from build123d import *

# Parameters (mm, degrees)
SKETCH1_R           = 39.751
BOSS_EXTRUDE1_DEPTH = 103.124
SKETCH2_R           = 17.4625
BOSS_EXTRUDE2_DEPTH = 2.54
SKETCH3_R           = 6.35
BOSS_EXTRUDE3_DEPTH = 41.91
BOSS_EXTRUDE4_START = 14.224
SKETCH4_R           = 6.35
BOSS_EXTRUDE4_DEPTH = 14.224
SKETCH5_R           = 1.999996
CUT_EXTRUDE1_DEPTH  = 6.858


with BuildPart() as part:
    # Sketch1 → Boss-Extrude1 (new body)
    with BuildSketch(Plane(origin=(0, 0, 0), x_dir=(0, 0, -1), z_dir=(1, 0, 0))):
        Circle(SKETCH1_R)
    extrude(amount=BOSS_EXTRUDE1_DEPTH)

    # Sketch2 → Boss-Extrude2 (add)
    with BuildSketch(Plane(origin=(103.124, 0, 0), x_dir=(0, 0, -1), z_dir=(1, 0, 0))):
        Circle(SKETCH2_R)
    extrude(amount=BOSS_EXTRUDE2_DEPTH)

    # Sketch3 → Boss-Extrude3 (add)
    with BuildSketch(Plane(origin=(105.664, 0, 0), x_dir=(0, 0, -1), z_dir=(1, 0, 0))):
        Circle(SKETCH3_R)
    extrude(amount=BOSS_EXTRUDE3_DEPTH)

    # Sketch4 → Boss-Extrude4 (add)
    with BuildSketch(Plane.ZY.offset(BOSS_EXTRUDE4_START)):
        with Locations(Location((0, 0, 0), (0, 0, 180))):
            Circle(SKETCH4_R)
    extrude(amount=-BOSS_EXTRUDE4_DEPTH)

    # Sketch5 → Cut-Extrude1 (cut)
    with BuildSketch(Plane(origin=(103.124, 0, 0), x_dir=(0, 0, -1), z_dir=(1, 0, 0))):
        with Locations((-14.882420075, 20.086004442)):
            Circle(SKETCH5_R)
        with Locations((20.086004442, 14.882420075)):
            Circle(SKETCH5_R)
        with Locations((14.882420075, -20.086004442)):
            Circle(SKETCH5_R)
        with Locations((-20.086004442, -14.882420075)):
            Circle(SKETCH5_R)
    extrude(amount=-CUT_EXTRUDE1_DEPTH, mode=Mode.SUBTRACT)


solid = part.part
Check sheet for the modelled part. Datum: model origin and axes. Units: mm. A direction names the side the tool comes from. Round coordinates to 2 decimals unless told otherwise and drop trailing zeros. Order: outer loops, then holes, each group sorted by start corner. A loop starts at its lowest first (then second) coordinate and runs counter-clockwise, first axis right, second up. Notation, with made-up numbers: M -37.75,20 L 13.25,20 A28 cw 13.25,59 Z; hole C 3,63.25 d3. An arc over 180 degrees is marked long. One line per item, written item: value. Start each with the question number.
1. Section check D-D on x = 125.5. Enter the section's corners in (y, z).
2. Section check A-A on y = 0. Enter the section's corners in (x, z), and give its area (3 significant figures).
3. Section check C-C on x = 78. Enter the section's corners in (y, z), and give its area (3 significant figures).
4. Release check for a two-part mould opening along Z. For faces 4 (the cylindrical face through (50.84, -38.806, 8.617)), 5 (the cylindrical face through (99.743, 14.97, -18.088)), 6 (the flat face through (0, 1, -8)) record: released by +Z, released by -Z, zero draft, split by the parting line, or undercut.
5. Access from +Z, -Z, +X, -X, +Y, -Y to the whole of each face (thin tool, end or side, straight path). Record for faces 1 (the flat face through (-14.224, 0, 0)), 2 (the cylindrical face through (-7.212, 5.634, -2.93)), 3 (the flat face through (96.266, -15, 20)).
6. Scan lines: line 1 along X through (y, z) = (-14, 8); line 2 along Y through (x, z) = (103, -14.5); line 3 along X through (y, z) = (8, 25). Record each from-to range of solid material in increasing order.
7. Gauge pin test, flat ends, axial feed: P1, Ø8, axis at y = -15, z = -29, coming from the +X side; P2, Ø1.2, axis at y = 20, z = 15.5, coming from the +X side; P3, Ø10, axis at y = -25, z = 30, coming from the -X side. Record the tip position at first contact, or that the pin passes through.
Results found:
1. outline: C 0,0 d12.7
2. outline: M -14.22,-6.35 L 0,-6.35 L 0,-39.75 L 103.12,-39.75 L 103.12,-17.46 L 105.66,-17.46 L 105.66,-6.35 L 147.57,-6.35 L 147.57,6.35 L 105.66,6.35 L 105.66,17.46 L 103.12,17.46 L 103.12,39.75 L 0,39.75 L 0,6.35 L -14.22,6.35 Z
2. area: 9,000 mm^2
3. outline: C 0,0 d79.5
3. area: 4,960 mm^2
4. face 4: split by the parting line
4. face 5: undercut
4. face 6: zero draft
5. face 1: +Z, -Z, -X, +Y, -Y
5. face 2: -X
5. face 3: +X
6. line 1: 0 to 105.66
6. line 2: -37.01 to -22.05, -18.12 to 37.01
6. line 3: 0 to 103.12
7. P1: x = 103.12
7. P2: x = 96.27
7. P3: x = 0
